Autodesk Inventor part; units mm, degrees
ref_plane "YZ Plane" through (0, 0, 0) normal (1, 0, 0) x (0, 1, 0)
ref_plane "XZ Plane" through (0, 0, 0) normal (0, 1, 0) x (-1, 0, 0)
ref_plane "XY Plane" through (0, 0, 0) normal (0, 0, 1) x (1, 0, 0)
sketch "Sketch1" plane through (0, 0, 0) normal (0, 0, 1) x (1, 0, 0)
  line L0 (-4.8, 0) -> (0.8, 0) construction
  line L1 (0, -38.15) -> (0, 38.15) construction
  line L2 (-4, 27.25) -> (0, 27.25)
  line L3 (0, 27.25) -> (0, -27.25)
  line L4 (0, -27.25) -> (-4, -27.25)
  line L5 (-4, -27.25) -> (-4, 27.25)
  point P0 (0, 0)
  dimension "d1" = 54.5
  dimension "d16" = 8
revolve "Revolution1" add sketch "Sketch1" angle 360 about axis through (0, -10, 0) along (0, 1, 0)
sketch "Sketch2" plane through (0, 27.25, 0) normal (0, 1, 0) x (1, 0, 0)
  circle A0 centre (0, 0) radius 4
hole "Hole1" at (0, 27.25, 0) direction (0, -1, 0) diameter 2.459 depth 15 tip angle 118
mirror "Espelhar1" [suppressed]
chamfer "Chamfer1" distance 0.5 angle 45 2 edges at (4, -27.25, 0) (4, 27.25, 0)
chamfer "Chamfer2" distance 0.3 angle 45 1 edges at (0, 27.25, -1.2295)
properties part number "GRJ-05-103" material "Poliacetal WT"
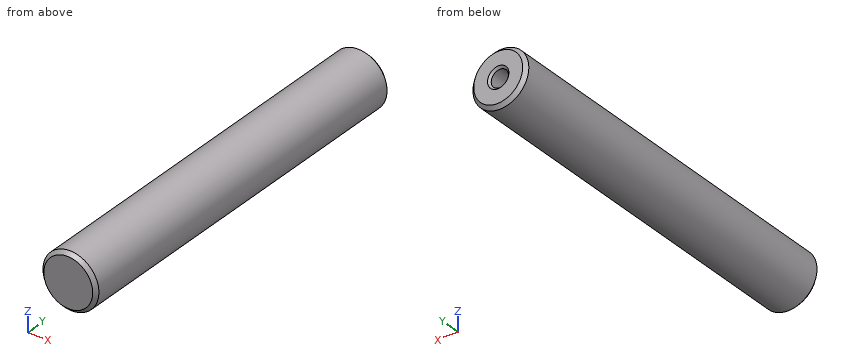
The model under review builds one solid part; all positions refer to its coordinate system, in mm. Round coordinates to 2 decimals unless told otherwise and drop trailing zeros. Order: outer loops, then holes, each group sorted by start corner. A loop starts at its lowest first (then second) coordinate and runs counter-clockwise, first axis right, second up. Notation, with made-up numbers: (66.25, 14.25) - (91.25, 14.25) arc R20 cw to (91.25, 47.25) - close; hole circle Ø3 at (-22.75, -32.5). An arc over 180 degrees is marked (long way). Answer in a Markdown table with one row per item.
(1) Take a section at A-A on y = -14. Write out the cut boundary in (x, z).
Result set:
| item | result |
|---|---|
| outline | circle Ø8 at (0, 0) |
(2) Take a section at B-B on y = 16. Write out the cut boundary in (x, z), plus the area to 3 significant figures.
Result set:
| item | result |
|---|---|
| outline | circle Ø8 at (0, 0); hole circle Ø2.46 at (0, 0) |
| area | 45.5 mm2 |
(3) For line 1 (Z direction, x = 0, y = 23); line 2 (Z direction, x = 0.75, y = 24.5); line 3 (Y direction, x = -1.5, z = -3.25), list the stretches that pass through material, from the lowest coordinate up. Write a range as from..to.
Result set:
| item | result |
|---|---|
| line 1 | z = -4..-1.23, 1.23..4 |
| line 2 | z = -3.93..-0.97, 0.97..3.93 |
| line 3 | y = -27.17..27.17 |
(4) Clearance check with a flat-ended pin moving along its axis: P1, Ø2, axis at x = -3, y = -7, coming from the -Z side. State where the tip first meets the part, or that it passes through.
Result set:
| item | result |
|---|---|
| P1 | stops at z = -3.46 |
